Work out the finished part from the listing and answer in its coordinate system (mm). Face numbers are marked on the shaded views. A direction names the side the tool comes from. Coordinates: 2 decimals unless noted, no trailing zeros. Order: outer loops, then holes, each group sorted by start corner. A loop starts at its lowest first (then second) coordinate and runs counter-clockwise, first axis right, second up. Notation, with made-up numbers: M -35,57 L -16,57 A12 cw -16,70 Z; hole C -25.75,-24.5 d3. An arc over 180 degrees is marked long. Write item = value, one per line. Start each with the question number.
Q1. Find section C-C on x = -0.25. Give the vertices of the cut face in (y, z), and give its area (3 significant figures).
Q2. Find section D-D on z = 13.25. Give the vertices of the cut face in (x, y).
Q3. Straight lines are drawn through the part: line 1 along Y through (x, z) = (0, 1.3); line 2 along Z through (x, y) = (-6, 1); line 3 along X through (y, z) = (-7.5, 3.25). For each, find the intervals that lie inside material, in ascending order.
Q4. Determine the mould class of the marked faces 1, 2 and 3 for opening direction X: released by +X, released by -X, zero draft, split by the parting line, or undercut.
Q5. Each of these flat-tipped pins is pushed along its axis until it touches: P1, Ø2.5, axis at x = 0, z = 11.5, coming from the +Y side; P2, Ø3, axis at x = 7.08, y = -0.01, coming from the +Z side; P3, Ø8, axis at y = -5, z = 8, coming from the +X side; P4, Ø1.9, axis at x = 0.09, y = -7.18, coming from the +Z side. Where does it stop, or does it pass through?
Q6. Find section A-A on x = 6.25. Give the vertices of the cut face in (y, z).
Q7. Find section B-B on y = -0.5. Give the vertices of the cut face in (x, z), and give its area (3 significant figures).
Q8. A tool of negligible diameter and unlimited length cuts with its end or side. For the marked faces 4, 5 and 6, from which of +Z, -Z, +X, -X, +Y, -Y can it reach the whole face along a straight path? Write none if from no direction.
```python
from build123d import *

# Parameters (mm, degrees)
ESQUISSE1_R                  = 10
BOSS_EXTRU_1_DEPTH           = 3.91
D_GAGEMENT_M21_D             = 2.4
R_P_TITION_CIRCULAIRE1_COUNT = 4
ESQUISSE4_R                  = 3
BOSS_EXTRU_2_DEPTH           = 10
ESQUISSE5_W                  = 6
ESQUISSE5_H                  = 1.22
ENL_V_MAT_EXTRU_1_DEPTH      = 10
ESQUISSE6_R                  = 4
ENL_V_MAT_EXTRU_2_DEPTH      = 1.91


with BuildPart() as part:
    # Esquisse1 → Boss.-Extru.1 (new body)
    with BuildSketch(Plane.XY):
        Circle(ESQUISSE1_R)
    extrude(amount=BOSS_EXTRU_1_DEPTH)

    # Dégagement M21 (through all)
    with Locations(Plane(origin=(-0.088339646, 6.978832002, 3.91), x_dir=(1, 0, 0), z_dir=(0, 0, 1))):
        with Locations((0, 0)):
            d_gagement_m21 = Hole(D_GAGEMENT_M21_D / 2)

    # Répétition circulaire1: Dégagement M21 ×4 about axis
    r_p_tition_circulaire1_axis = Axis((0.001290677, -0.101963455, 0), (0, 0, 1))
    for i in range(1, R_P_TITION_CIRCULAIRE1_COUNT):
        add(d_gagement_m21.rotate(r_p_tition_circulaire1_axis, i * 360 / R_P_TITION_CIRCULAIRE1_COUNT), mode=Mode.SUBTRACT)

    # Esquisse4 → Boss.-Extru.2 (add)
    with BuildSketch(Plane.XY.offset(3.91)):
        Circle(ESQUISSE4_R)
    extrude(amount=BOSS_EXTRU_2_DEPTH)

    # Esquisse5 → Enlèv. mat.-Extru.1 (cut)
    with BuildSketch(Plane.XY.offset(13.91)):
        with Locations((0, 2.39)):
            Rectangle(ESQUISSE5_W, ESQUISSE5_H)
    extrude(amount=-ENL_V_MAT_EXTRU_1_DEPTH, mode=Mode.SUBTRACT)

    # Esquisse6 → Enlèv. mat.-Extru.2 (cut)
    with BuildSketch(Plane(origin=(0, 0, 0), x_dir=(-1, 0, 0), z_dir=(0, 0, -1))):
        Circle(ESQUISSE6_R)
    extrude(amount=-ENL_V_MAT_EXTRU_2_DEPTH, mode=Mode.SUBTRACT)


solid = part.part
```
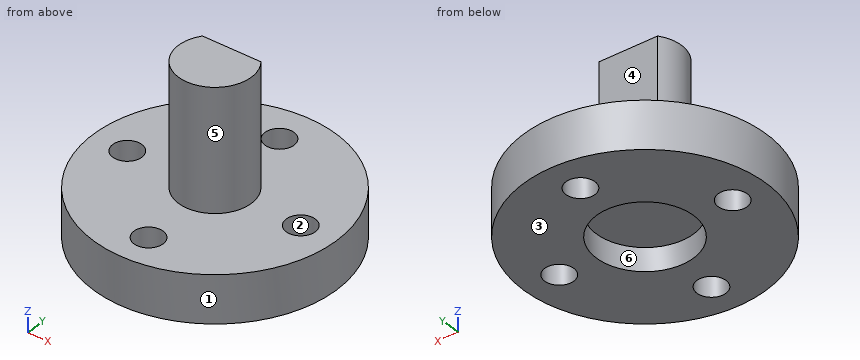
Findings below:
q1.outline = M -10,0 L -8.33,0 L -8.33,3.91 L -10,3.91 Z; M -6.03,0 L -3.99,0 L -3.99,1.91 L 3.99,1.91 L 3.99,0 L 5.79,0 L 5.79,3.91 L 1.78,3.91 L 1.78,13.91 L -2.99,13.91 L -2.99,3.91 L -6.03,3.91 Z; M 8.17,0 L 10,0 L 10,3.91 L 8.17,3.91 Z
q1.area = 92.3 mm^2
q2.outline = M -2.41,1.78 A3 ccw long 2.41,1.78 Z
q3.line_1 = -10 to -8.38, -5.99 to -4, 4 to 5.78, 8.18 to 10
q3.line_2 = 0 to 3.91
q3.line_3 = -6.61 to -1.07, 1.25 to 6.61
q4.face_1 = split by the parting line
q4.face_2 = undercut
q4.face_3 = zero draft
q5.P1 = 1.78
q5.P2 = 3.91
q5.P3 = 2.83
q5.P4 = through
q6.outline = M -7.81,0 L -0.88,0 L -0.88,3.91 L -7.81,3.91 Z; M 0.85,0 L 7.81,0 L 7.81,3.91 L 0.85,3.91 Z
q7.outline = M -9.99,0 L -8.24,0 L -8.24,3.91 L -9.99,3.91 Z; M -5.92,0 L -3.97,0 L -3.97,1.91 L 3.97,1.91 L 3.97,0 L 5.99,0 L 5.99,3.91 L 2.96,3.91 L 2.96,13.91 L -2.96,13.91 L -2.96,3.91 L -5.92,3.91 Z; M 8.18,0 L 9.99,0 L 9.99,3.91 L 8.18,3.91 Z
q7.area = 104 mm^2
q8.face_4 = +Z, +X, -X, +Y
q8.face_5 = +Z
q8.face_6 = -Z
